Build history of the part. All positions in model axes, mm. Round coordinates to 2 decimals unless told otherwise and drop trailing zeros. Write each loop counter-clockwise with the first axis right and the second up, starting at its lowest first coordinate (ties: lowest second). Pieces come first, ordered by that corner, then holes. Notation, with made-up numbers: (-39.75, -33) -> (-23.75, -33) arc R30 cw to (-23.75, -1) -> close; hole circle Ø5 at (13.5, 81). An arc over 180 degrees is marked (long way). Return JSON: item names as keys, results as strings.
from build123d import *

# Parameters (mm, degrees)
SKETCH022_W         = 115
SKETCH022_H         = 78
PAD010_DEPTH        = 3
HOLE002_D           = 3.4
HOLE002_DEPTH       = 5
HOLE002_CSINK_D     = 6.1
HOLE002_CSINK_ANGLE = 90
SKETCH027_W         = 29
SKETCH027_H         = 29
POCKET009_DEPTH     = 1
CHAMFER001_SIZE     = 0.75


with BuildPart() as part:
    # Sketch022 (on Face1 of CopyPad011) → Pad010 (new body)
    with BuildSketch(Plane.XY.offset(24)):
        with Locations((52.5, 32)):
            Rectangle(SKETCH022_W, SKETCH022_H)
    extrude(amount=PAD010_DEPTH)

    # Hole002
    with Locations(Plane.XY.offset(27)):
        with Locations((-1, 67), (106, 67), (106, -3), (-1, -3), (32, 67), (73, -3), (32, -3), (73, 67)):
            CounterSinkHole(HOLE002_D / 2, HOLE002_CSINK_D / 2, depth=HOLE002_DEPTH, counter_sink_angle=HOLE002_CSINK_ANGLE)

    # Sketch027 → Pocket009 (cut)
    with BuildSketch(Plane(origin=(0, 0, 24), x_dir=(1, 0, 0), z_dir=(0, 0, -1))):
        with Locations((27.5, -16.5)):
            Rectangle(SKETCH027_W, SKETCH027_H)
    extrude(amount=-POCKET009_DEPTH, mode=Mode.SUBTRACT)

    # Chamfer001
    chamfer001_edges = [part.edges().sort_by_distance(p)[0] for p in [
        (52.5, 71, 27),
        (110, 71, 25.5),
        (110, 32, 27),
        (52.5, -7, 27),
        (110, -7, 25.5),
        (-5, 32, 27),
        (-5, 71, 25.5),
        (-5, -7, 25.5),
    ]]
    chamfer(chamfer001_edges, length=CHAMFER001_SIZE)


with BuildPart() as part_1:
    # Body002 placement: moved
    add(part.part.moved(Location((0, 0, -2.5))))


solid = part_1.part
Q1. Saw through at A-A on y = -3. Count the separate pieces of the cut face and the enclosed holes in it, then the cut area to 3 significant figures.
Verdict:
{"separate pieces": "5", "enclosed holes": "0", "area": "296 mm²"}
Q2. Two-plate mould, pull along X, no slides. Class faces 1 (the flat face through (110, 31, 23)), 2 (the cylindrical face through (107.7, -2.93, 22.31)), 3 (the flat face through (-5, 31, 23)): +X half, -X half, draft (parallel to the pull), parting line (faces both ways), or undercut.
Verdict:
{"face 1": "+X half", "face 2": "undercut", "face 3": "-X half"}
Q3. Pin check, flat tips, straight feed: pin 1 Ø4.5 at (x, y) = (106, -3) entering from +Z; pin 2 Ø1 at (y, z) = (59.5, 24) entering from -X; pin 3 Ø5.5 at (x, y) = (32, 67) entering from +Z. Stop position of each tip, or through.
Verdict:
{"pin 1": "stops at z = 23.7", "pin 2": "stops at x = -5", "pin 3": "stops at z = 24.2"}
Q4. Wall check: L1, parallel to X at y = -3, z = 22.8; L2, parallel to Y at x = -1, z = 22.3; L3, parallel to Y at x = 22, z = 22.35. Give the ranges that are in metal, low to high.
Verdict:
{"L1": "x = -5 to -2.7, 0.7 to 30.3, 33.7 to 71.3, 74.7 to 104.3, 107.7 to 110", "L2": "y = -7 to -4.7, -1.3 to 65.3, 68.7 to 71", "L3": "y = -7 to 2, 31 to 71"}
Q5. Saw through at D-D on x = 19.5. List the corners of the cut face in (y, z).
Verdict:
{"outline": "(-7, 21.5) -> (2, 21.5) -> (2, 22.5) -> (31, 22.5) -> (31, 21.5) -> (71, 21.5) -> (71, 23.75) -> (70.25, 24.5) -> (-6.25, 24.5) -> (-7, 23.75) -> close"}
Q6. Saw through at B-B on x = 106. List the corners of the cut face in (y, z).
Verdict:
{"outline": "(-7, 21.5) -> (-4.7, 21.5) -> (-4.7, 23.15) -> (-6.05, 24.5) -> (-6.25, 24.5) -> (-7, 23.75) -> close; (-1.3, 21.5) -> (65.3, 21.5) -> (65.3, 23.15) -> (63.95, 24.5) -> (0.05, 24.5) -> (-1.3, 23.15) -> close; (68.7, 21.5) -> (71, 21.5) -> (71, 23.75) -> (70.25, 24.5) -> (70.05, 24.5) -> (68.7, 23.15) -> close"}
Q7. Saw through at C-C on y = 6. List the corners of the cut face in (x, z), then the cut area to 3 significant figures.
Verdict:
{"outline": "(-5, 21.5) -> (13, 21.5) -> (13, 22.5) -> (42, 22.5) -> (42, 21.5) -> (110, 21.5) -> (110, 23.75) -> (109.25, 24.5) -> (-4.25, 24.5) -> (-5, 23.75) -> close", "area": "315 mm²"}
